Here's how the part is built. I have some questions about the finished solid (model axes, mm). A direction names the side the tool comes from. Coordinates: 2 decimals unless noted, no trailing zeros. Loops run counter-clockwise (first coordinate to the right, second up) from the corner with the lowest first, then second, coordinate; pieces in that order, holes last. Notation, with made-up numbers: M -2.5,2 L 20.5,2 A28 ccw 20.5,20 Z; hole C -1.5,-35 d2. An arc over 180 degrees is marked long. Use one line per item in the form item = value. Start each with the question number.
(1) On a 3-axis mill with a long thin cutter (end or side, diameter ignored), from which of +Z, -Z, +X, -X, +Y, -Y can I reach the whole of each face in a straight line? I mean faces 5 (the flat face through (10, -2.5, 54)), 6 (the flat face through (10, -5, 47)), 7 (the cylindrical face through (-14.985, 0.66, 13.599)). Say none if no direction works.
(2) Thinking about a two-plate mould opening in Z: for faces 1 (the cylindrical face through (-2.38, -10.74, 48.01)), 2 (the flat face through (-11, 7, 25)), 3 (the flat face through (-11, -3, 49)), 4 (the flat face through (0, 0, 0)), which applies, +Z half, -Z half, draft (parallel to the pull), parting line (faces both ways), or undercut?
(3) Imagine slicing it at C-C, the plane z = 48. Please give me the cut outline in (x, y).
(4) Will these pins go through, and if not, where does the flat tip stop? P1, Ø3, axis at y = 3, z = 48, coming from the +X side; P2, Ø4, axis at x = -12.5, z = 15.5, coming from the +Y side; P3, Ø2, axis at y = -5, z = 20, coming from the -X side; P4, Ø4, axis at x = -3, y = 12, coming from the -Z side.
(5) Imagine slicing it at B-B, the plane z = 17.5. Please give me the cut outline in (x, y).
(6) Please list where these lines run through material, in increasing order: L1, parallel to Z at x = 0, y = -15.5; L2, parallel to X at y = -3.5, z = 36.
```python
from build123d import *

# Parameters (mm, degrees)
SKETCH_1_R          = 17.45
EXTRUDE_1_DEPTH     = 3
SKETCH_2_R          = 15
EXTRUDE_2_DEPTH     = 22
SKETCH_4_R          = 12.5
EXTRUDE_3_DEPTH     = 22
SKETCH_5_R          = 12
EXTRUDE_4_DEPTH     = 12
CHAMFER_1_SIZE      = 0.5
SKETCH_6_W          = 1
SKETCH_6_H          = 2
CHAMFER_2_SIZE      = 0.5
CHAMFER_3_SIZE      = 1
SKETCH_7_W          = 12
SKETCH_7_H          = 5
CUT_EXTRUDE_1_DEPTH = 3
FILLET_1_R          = 2.5


with BuildPart() as part:
    # 草图1 → 拉伸1 (new body)
    with BuildSketch(Plane.XY):
        Circle(SKETCH_1_R)
    extrude(amount=EXTRUDE_1_DEPTH)

    # 草图2 → 拉伸2 (add)
    with BuildSketch(Plane.XY.offset(3)):
        Circle(SKETCH_2_R)
    extrude(amount=EXTRUDE_2_DEPTH)

    # 草图4 → 拉伸3 (add)
    with BuildSketch(Plane.XY.offset(25)):
        Circle(SKETCH_4_R)
    extrude(amount=EXTRUDE_3_DEPTH)

    # 草图5 → 拉伸4 (add)
    with BuildSketch(Plane.XY.offset(47)):
        Circle(SKETCH_5_R)
    extrude(amount=EXTRUDE_4_DEPTH)

    # 倒角1
    chamfer_1_edges = [part.edges().sort_by_distance(p)[0] for p in [
        (-12, 0, 59),
    ]]
    chamfer(chamfer_1_edges, length=CHAMFER_1_SIZE)

    # 草图6 → 切除-旋转1 (revolve, cut)
    with BuildSketch(Plane(origin=(0, 0, 0), x_dir=(1, 0, 0), z_dir=(0, 1, 0)), mode=Mode.PRIVATE) as cut_revolve_1_sk:
        with Locations((-11.5, -48)):
            Rectangle(SKETCH_6_W, SKETCH_6_H)
    revolve(cut_revolve_1_sk.sketch.rotate(Axis((0, 0, 47), (0, 0, -1)), 180), axis=Axis((0, 0, 47), (0, 0, -1)), mode=Mode.SUBTRACT)

    # 倒角2
    chamfer_2_edges = [part.edges().sort_by_distance(p)[0] for p in [
        (-12.5, 0, 47),
        (-17.45, 0, 3),
        (-15, 0, 25),
    ]]
    chamfer(chamfer_2_edges, length=CHAMFER_2_SIZE)

    # 倒角3
    chamfer_3_edges = [part.edges().sort_by_distance(p)[0] for p in [
        (-17.45, 0, 0),
    ]]
    chamfer(chamfer_3_edges, length=CHAMFER_3_SIZE)

    # 草图7 → 切除-拉伸1 (cut)
    with BuildSketch(Plane(origin=(12, 0, 0), x_dir=(0, 0, -1), z_dir=(1, 0, 0))):
        with Locations((-53, 0)):
            Rectangle(SKETCH_7_W, SKETCH_7_H)
    extrude(amount=-CUT_EXTRUDE_1_DEPTH, mode=Mode.SUBTRACT)

    # 圆角1
    # the kernel refuses this fillet: 2.5 mm, written as the material it adds along each edge
    with BuildSketch(Plane(origin=(16.962142643, -2.5, 47), x_dir=(0, 1, 0), z_dir=(-1, 0, 0))) as fillet_1_piece_1_section:
        with BuildLine():
            CenterArc((FILLET_1_R, -FILLET_1_R), FILLET_1_R, 90, 90)
            Line((0, -FILLET_1_R), (0, 0))
            Line((0, 0), (FILLET_1_R, 0))
        make_face()
    fillet_1_piece_1 = extrude(amount=14.212142643, mode=Mode.PRIVATE)
    fillet_1_piece_1 = fillet_1_piece_1 & Plane(origin=(0, 0, 49.124758418), x_dir=(1, 0, 0), z_dir=(0, 0, -1)) * Cylinder(12, 39, mode=Mode.PRIVATE)
    fillet_1_piece_1 = split(fillet_1_piece_1, bisect_by=Plane(origin=(11.227777132, -2.484876178, 49), z_dir=(0, 0, 1)), keep=Keep.TOP, mode=Mode.PRIVATE)
    add(fillet_1_piece_1)
    with BuildSketch(Plane(origin=(16.962142643, -2.5, 47), x_dir=(0, 1, 0), z_dir=(-1, 0, 0))) as fillet_1_piece_2_section:
        with BuildLine():
            CenterArc((FILLET_1_R, -FILLET_1_R), FILLET_1_R, 90, 90)
            Line((0, -FILLET_1_R), (0, 0))
            Line((0, 0), (FILLET_1_R, 0))
        make_face()
    fillet_1_piece_2 = extrude(amount=14.212142643, mode=Mode.PRIVATE)
    fillet_1_piece_2 = fillet_1_piece_2 & Plane(origin=(0, 0, 48.528388409), x_dir=(1, 0, 0), z_dir=(0, 0, 1)) * Cylinder(11, 39, mode=Mode.PRIVATE)
    add(fillet_1_piece_2)
    with BuildSketch(Plane(origin=(16.962142643, 2.5, 47), x_dir=(0, -1, 0), z_dir=(-1, 0, 0))) as fillet_1_piece_3_section:
        with BuildLine():
            CenterArc((FILLET_1_R, FILLET_1_R), FILLET_1_R, 180, 90)
            Line((0, FILLET_1_R), (0, 0))
            Line((0, 0), (FILLET_1_R, 0))
        make_face()
    fillet_1_piece_3 = extrude(amount=14.212142643, mode=Mode.PRIVATE)
    fillet_1_piece_3 = fillet_1_piece_3 & Plane(origin=(0, 0, 49.124758418), x_dir=(1, 0, 0), z_dir=(0, 0, -1)) * Cylinder(12, 39, mode=Mode.PRIVATE)
    fillet_1_piece_3 = split(fillet_1_piece_3, bisect_by=Plane(origin=(11.227777136, 2.484876178, 49), z_dir=(0, 0, 1)), keep=Keep.TOP, mode=Mode.PRIVATE)
    add(fillet_1_piece_3)
    with BuildSketch(Plane(origin=(16.962142643, 2.5, 47), x_dir=(0, -1, 0), z_dir=(-1, 0, 0))) as fillet_1_piece_4_section:
        with BuildLine():
            CenterArc((FILLET_1_R, FILLET_1_R), FILLET_1_R, 180, 90)
            Line((0, FILLET_1_R), (0, 0))
            Line((0, 0), (FILLET_1_R, 0))
        make_face()
    fillet_1_piece_4 = extrude(amount=14.212142643, mode=Mode.PRIVATE)
    fillet_1_piece_4 = fillet_1_piece_4 & Plane(origin=(0, 0, 48.5283884), x_dir=(1, 0, 0), z_dir=(0, 0, 1)) * Cylinder(11, 39, mode=Mode.PRIVATE)
    add(fillet_1_piece_4)


solid = part.part
```
Answer:
q1.face_5 = +Z, +X
q1.face_6 = none
q1.face_7 = +Z
q2.face_1 = undercut
q2.face_2 = +Z half
q2.face_3 = undercut
q2.face_4 = -Z half
q3.outline = M 9,-2 L 9,2 L 10.82,2 A11 ccw long 10.82,-2 Z
q4.P1 = 12.17
q4.P2 = 10.71
q4.P3 = -14.46
q4.P4 = 0
q5.outline = C 0,0 d30
q6.L1 = 0 to 3
q6.L2 = -12 to 12
